Answer from the drawing. Dimensions are ordinates in mm from the lowest x, y and z of the part. Give positions to 0.01 mm unless a question says otherwise; leave off trailing zeros. Write each loop counter-clockwise with the first axis right and the second up, starting at its lowest first coordinate (ties: lowest second). Pieces come first, ordered by that corner, then holes. Notation, with made-up numbers: (-37, -9) - (-14, -9) arc R16 ccw to (-14, -2) - close; hole circle Ø11 at (-26.75, 53.5). An arc over 180 degrees is marked (long way). Write item = value, one per line.
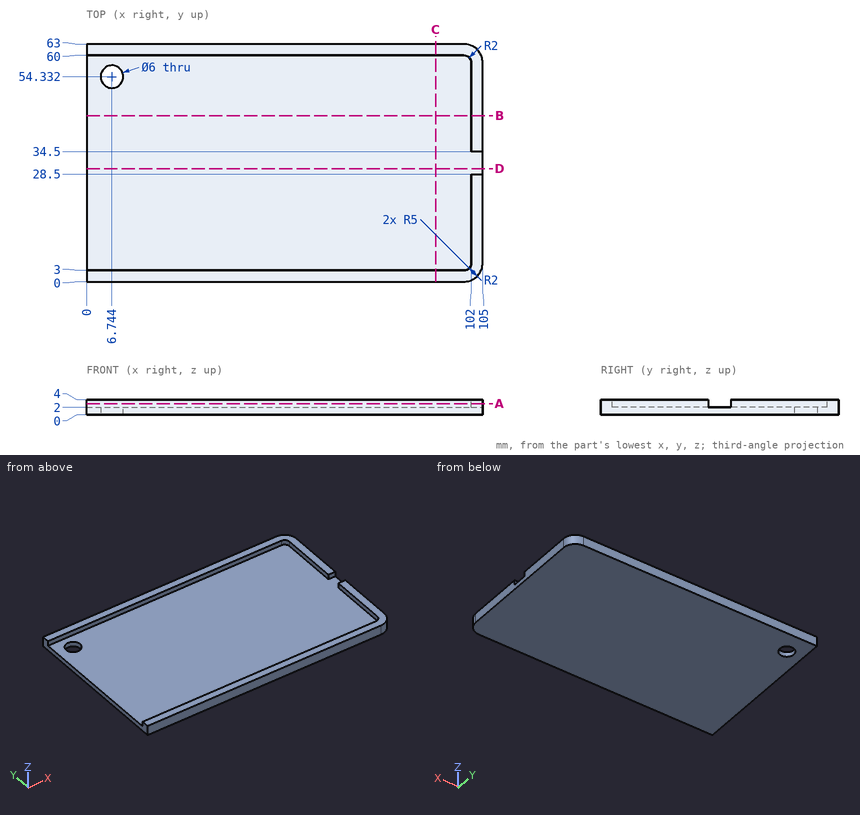
1. Given pin 1 (3.5 mm diameter, centred on x = 6.74, y = 54.33, fed in from -Z); pin 2 (17 mm diameter, centred on x = 72.5, y = 30.5, fed in from +Z); pin 3 (1 mm diameter, centred on y = 21, z = 3.5, fed in from -X); pin 4 (1 mm diameter, centred on x = 103.5, z = 3, fed in from +Y), each flat-ended and moving along its own axis, determine where each tip first touches the part or whether it passes through.
Solution:
pin_1 = through
pin_2 = 2
pin_3 = 102
pin_4 = 62
2. Find section C-C, the plane x = 92.5. Give the vertices of the cut face in (y, z).
Solution:
outline = (0, 0) - (63, 0) - (63, 4) - (60, 4) - (60, 2) - (3, 2) - (3, 4) - (0, 4) - close
3. Find section D-D, the plane y = 30. Give the vertices of the cut face in (x, z), then the cut area to 3 significant figures.
Solution:
outline = (0, 0) - (105, 0) - (105, 2) - (0, 2) - close
area = 210 mm^2
4. Straight lines are drawn through the part: line 1 (Y direction, x = 21, z = 3.55); line 2 (X direction, y = 36, z = 2.75); line 3 (Z direction, x = 78, y = 24). For each, find the intervals that lie inside material, in ascending order.
Solution:
line_1 = 0 to 3, 60 to 63
line_2 = 102 to 105
line_3 = 0 to 2
5. Find section A-A, the plane z = 2.95. Give the vertices of the cut face in (x, y), then the cut area to 3 significant figures.
Solution:
outline = (0, 0) - (100, 0) arc R5 ccw to (105, 5) - (105, 28.5) - (102, 28.5) - (102, 5) arc R2 cw to (100, 3) - (0, 3) - close; (0, 60) - (100, 60) arc R2 cw to (102, 58) - (102, 34.5) - (105, 34.5) - (105, 58) arc R5 ccw to (100, 63) - (0, 63) - close
area = 774 mm^2
6. Find section B-B, the plane y = 44. Give the vertices of the cut face in (x, z).
Solution:
outline = (0, 0) - (105, 0) - (105, 4) - (102, 4) - (102, 2) - (0, 2) - close
